```python
from build123d import *

# Parameters (mm, degrees)
BOSS_EXTRUDE1_DEPTH                              = 22.86
M3_CLEARANCE_HOLE1_D                             = 3.4
CBORE_FOR_M3_PAN_HEAD_MACHINE_SCREW1_D           = 3.4
CBORE_FOR_M3_PAN_HEAD_MACHINE_SCREW1_CBORE_D     = 7
CBORE_FOR_M3_PAN_HEAD_MACHINE_SCREW1_CBORE_DEPTH = 2.4
CUT_EXTRUDE1_DEPTH                               = 2.54


with BuildPart() as part:
    # Model → Boss-Extrude1 (new body)
    with BuildSketch(Plane.XY):
        Polygon((-31.561530074, 5.719031337), (-31.559190751, -16.756549884), (-29.679250105, -22.022082599), (-25.638762019, -26.336998537), (-19.362308162, -29.395591134), (-17.768021154, -29.956483893), (-16.704264105, -30.309706307), (-8.455081931, -32.518568858), (-1.9378711, -33.964713672), (0.686481117, -35.620494321), (0.686481117, -56.318132067), (7.036481117, -56.318132067), (7.036481117, -32.118649881), (0.516193039, -28.004809234), (-6.945353494, -26.349119844), (-14.880902119, -24.224238152), (-15.713611559, -23.947735506), (-16.909625113, -23.526960991), (-21.804194775, -21.141777435), (-24.142511039, -18.644643945), (-25.264614821, -15.501739308), (-25.266693071, 4.465531103), (-24.147092478, 7.603487204), (-21.804194775, 10.105513301), (-16.909625113, 12.490696857), (-15.713611559, 12.911471373), (-14.880902119, 13.187974018), (-6.945353494, 15.312855711), (0.516193039, 16.9685451), (7.036481117, 21.082385748), (7.036481117, 45.281867933), (0.686481117, 45.281867933), (0.686481117, 24.584230187), (-1.9378711, 22.928449538), (-8.455081931, 21.482304725), (-16.704264105, 19.273442173), (-17.768021154, 18.92021976), (-19.362308162, 18.359327), (-25.638762019, 15.300734404), (-29.684302801, 10.980422593), align=None)
    extrude(amount=BOSS_EXTRUDE1_DEPTH)

    # M3 Clearance Hole1 (through all)
    with Locations(Plane.ZY.offset(-0.686481117)):
        with Locations((5.08, 36.391867933), (17.78, 36.391867933), (5.08, -47.308730357), (17.78, -47.308730357)):
            Hole(M3_CLEARANCE_HOLE1_D / 2)

    # CBORE for M3 Pan Head Machine Screw1 (through all)
    with Locations(Plane(origin=(-25.266228013, -0.002629781, 0), x_dir=(0, 0, -1), z_dir=(0.999999995, 0.000104083, 0))):
        with Locations((-5.08, -5.564839092), (-17.78, -5.564839092)):
            CounterBoreHole(CBORE_FOR_M3_PAN_HEAD_MACHINE_SCREW1_D / 2, CBORE_FOR_M3_PAN_HEAD_MACHINE_SCREW1_CBORE_D / 2, CBORE_FOR_M3_PAN_HEAD_MACHINE_SCREW1_CBORE_DEPTH)

    # Sketch5 → Cut-Extrude1 (cut)
    with BuildSketch(Plane.ZY.offset(-0.686481117)):
        Polygon((17.78, -43.642556148), (14.605, -45.475643253), (14.605, -49.141817462), (17.78, -50.974904567), (20.955, -49.141817462), (20.955, -45.475643253), align=None)
        Polygon((5.08, -43.642556148), (1.905, -45.475643253), (1.905, -49.141817462), (5.08, -50.974904567), (8.255, -49.141817462), (8.255, -45.475643253), align=None)
        Polygon((17.78, 40.058042143), (14.605, 38.224955038), (14.605, 34.558780829), (17.78, 32.725693724), (20.955, 34.558780829), (20.955, 38.224955038), align=None)
        Polygon((5.08, 40.058042143), (1.905, 38.224955038), (1.905, 34.558780829), (5.08, 32.725693724), (8.255, 34.558780829), (8.255, 38.224955038), align=None)
    extrude(amount=-CUT_EXTRUDE1_DEPTH, mode=Mode.SUBTRACT)


solid = part.part
```
CAD build for the part. Positions are in the model's coordinates, mm. A direction names the side the tool comes from. Coordinates: 2 decimals unless noted, no trailing zeros. Order: outer loops, then holes, each group sorted by start corner. A loop starts at its lowest first (then second) coordinate and runs counter-clockwise, first axis right, second up. Notation, with made-up numbers: (-34, -38) - (-13, -38) arc R19 cw to (-13, -20) - close; hole circle Ø4 at (19, -0.5). An arc over 180 degrees is marked (long way). Use a Markdown table: item, result. Add a question column.
(1) Flat gauge pins, fed straight in: pin 1 (7 mm diameter, centred on y = 37.5, z = 5.5, fed in from -X); pin 2 (2 mm diameter, centred on y = -29.5, z = 5.5, fed in from +X); pin 3 (8 mm diameter, centred on x = -8.5, z = 14.5, fed in from -Y). Where does each tip first touch, or does it go through?
(2) Drill centre lines: line 1 along Y through (x, z) = (1, 14.75); line 2 along Y through (x, z) = (6.2, 17.78); line 3 along X through (y, z) = (31, 16.5). Where is each one in solid material? Low to high. Write a range as [from, to].
(3) Pull direction Y, two halves, no side cores. Call faces 5 (the face through (-5.151, 22.216, 11.27)), 6 (the face through (-0.644, -34.781, 11.27)), 7 (the face through (1.94, 39.13, 6.69)): +Y half, -Y half, draft (parallel to the pull), parting line (faces both ways), or undercut.
(4) Which spindle directions (+Z, -Z, +X, -X, +Y, -Y) get a long thin tool onto all of the face, cutting with end or side? Do faces 1 (the face through (0.686, 35, 11)), 2 (the face through (1.94, 33.63, 19.35)), 3 (the face through (-24.715, 6.013, 11.27)), 4 (the face through (-30.632, -19.352, 11.27)). Say none if no direction does.
(5) Saw through at B-B (x = -12.5). Give the cut face in (y, z), then the cut area to 3 significant figures.
(6) Saw through at A-A (x = -0.5). Give the cut face in (y, z), then the cut area to 3 significant figures.
(7) Saw through at C-C (y = 3.5). Give the cut face in (x, z), then the cut area to 3 significant figures.
Solved:
| question | item | result |
|---|---|---|
| 1 | pin 1 | stops at x = 0.69 |
| 1 | pin 2 | stops at x = 4.47 |
| 1 | pin 3 | stops at y = -33.4 |
| 2 | line 1 | y = [-56.32, -49.23], [-45.39, -28.31], [17.27, 34.48], [38.31, 45.28] |
| 2 | line 2 | y = [-56.32, -49.01], [-45.61, -31.59], [20.55, 34.69], [38.09, 45.28] |
| 2 | line 3 | x = [0.69, 7.04] |
| 3 | face 5 | +Y half |
| 3 | face 6 | -Y half |
| 3 | face 7 | undercut |
| 4 | face 1 | +Z, -Z, -X, +Y |
| 4 | face 2 | -X |
| 4 | face 3 | +Z, -Z, +X |
| 4 | face 4 | +Z, -Z, -X, -Y |
| 5 | outline | (-31.44, 0) - (-24.86, 0) - (-24.86, 22.86) - (-31.44, 22.86) - close; (13.83, 0) - (20.4, 0) - (20.4, 22.86) - (13.83, 22.86) - close |
| 5 | area | 301 mm² |
| 6 | outline | (-34.87, 0) - (-27.78, 0) - (-27.78, 22.86) - (-34.87, 22.86) - close; (16.74, 0) - (23.84, 0) - (23.84, 22.86) - (16.74, 22.86) - close |
| 6 | area | 324 mm² |
| 7 | outline | (-31.56, 0) - (-25.27, 0) - (-25.27, 22.86) - (-31.56, 22.86) - close |
| 7 | area | 144 mm² |
